Geometry: final body of the model. Coordinates: model frame, mm. A direction names the side the tool comes from. Give positions to 0.01 mm unless a question says otherwise; leave off trailing zeros. Order: outer loops, then holes, each group sorted by start corner. A loop starts at its lowest first (then second) coordinate and runs counter-clockwise, first axis right, second up. Notation, with made-up numbers: (39.25, 39.25) - (94.25, 39.25) arc R32 cw to (94.25, 68.25) - close; hole circle Ø5 at (13, 77.25). An arc over 180 degrees is marked (long way). Use one line per item in the form item = value.
Autodesk Inventor part; units mm, degrees
ref_plane "Work Plane1" through (19.939, 0, 0) normal (1, 0, 0) x (0, 0, -1)
ref_plane "fan interface" through (0, 0, 5.3975) normal (0, 0, 1) x (1, 0, 0)
ref_plane "YZ Plane" through (0, 0, 0) normal (1, 0, 0) x (0, 1, 0)
sketch "Sketch1" plane through (0, 0, 0) normal (0, 0, 1) x (1, 0, 0)
  line L0 (0, 0) -> (39.878, 0)
  line L1 (39.878, 0) -> (39.878, 39.878)
  line L2 (39.878, 39.878) -> (0, 39.878)
  line L3 (0, 39.878) -> (0, 0)
  dimension "d0" = 39.878
  dimension "d1" = 39.878
extrude "Extrusion1" add sketch "Sketch1" along normal blind 19.812
ref_plane "Work Plane1" through (19.939, 0, 0) normal (1, 0, 0) x (0, 0, -1)
sketch "Sketch2" plane through (19.939, 0, 0) normal (1, 0, 0) x (0, 0, -1)
  line L0 (-19.812, 39.878) -> (-19.812, 0)
  line L1 (0, 0) -> (0, 39.878)
  line L2 (-19.812, 19.939) -> (0, 19.939)
  line L3 (-18.1102, 52.578) -> (-1.7018, 52.578)
  line L4 (-1.7018, 52.578) -> (-1.7018, 39.878)
  line L5 (-1.7018, 39.878) -> (-18.1102, 39.878)
  line L6 (-18.1102, 39.878) -> (-18.1102, 52.578)
  line L7 (-19.812, 39.878) -> (0, 39.878)
  dimension "d4" = 1.7018
  dimension "d5" = 1.7018
  dimension "d6" = 12.7
revolve "Revolution1" cut sketch "Sketch2" angle 360 about axis through (19.939, 19.939, 19.812) along (0, 0, -1) contours L6 L3 L4 L5
fillet "Fillet1" radius 3.175 7 edges at (39.878, 39.878, 18.9611) (39.878, 39.878, 0.8509) (0, 39.878, 18.9611) (0, 39.878, 0.8509) (0, 0, 0.8509) (39.878, 0, 0.8509) (39.878, 0, 18.9611)
sketch "Sketch3" plane through (0, 0, 19.812) normal (0, 0, 1) x (1, 0, 0)
  arc A0 (39.878, 36.703) -> (36.703, 39.878) centre (36.703, 36.703) ccw
  circle A1 centre (36.703, 36.703) radius 2.286
  dimension "d9" = 4.572
extrude "Extrusion2" cut sketch "Sketch3" against normal through all
sketch "Sketch4" plane through (19.939, 39.878, 1.7018) normal (0, 0, 1) x (1, 0, 0)
  circle A0 centre (16.764, -3.175) radius 2.286
  arc A1 (19.939, -3.175) -> (16.764, 0) centre (16.764, -3.175) ccw
  arc A2 (19.939, -19.939) -> (0, 0) centre (0, -19.939) ccw
  line L0 (16.764, -3.175) -> (0, -19.939)
  circle A3 centre (16.764, -3.175) radius 2.7094
  line L1 (18.6798, -5.0908) -> (15.8841, -7.8866)
  line L2 (14.8482, -1.2592) -> (12.0524, -4.0549)
extrude "Extrusion3" add sketch "Sketch4" along normal up to next
pattern_circular "Circular Pattern1" count 4 over 360 about axis through (19.939, 19.939, 9.906) along (0, 0, 1) of "Extrusion2", "Extrusion3"
sketch "Sketch5" plane through (0, 0, 19.812) normal (0, 0, 1) x (1, 0, 0)
  arc A0 (19.939, 39.878) -> (7.8866, 35.8231) centre (19.939, 19.939) ccw
  arc A1 (31.9914, 35.8231) -> (19.939, 39.878) centre (19.939, 19.939) ccw
  arc A2 (31.9914, 35.8231) -> (19.939, 39.878) centre (19.939, 19.939) ccw
  arc A3 (19.939, 39.878) -> (7.8866, 35.8231) centre (19.939, 19.939) ccw
  circle A4 centre (19.939, 19.939) radius 19.2405
  dimension "d19" = 38.481
extrude "Extrusion4" cut sketch "Sketch5" against normal through all
sketch "Sketch6" plane through (0, 0, 0) normal (0, 0, -1) x (-1, 0, 0)
  circle A0 centre (-19.939, 19.939) radius 19.2405
  circle A1 centre (-36.703, 3.175) radius 2.286
  line L0 (-15.6996, 8.562) -> (-35.9048, 1.0329)
  line L1 (-19.5524, 7.804) -> (-34.6449, 2.18)
  line L2 (-12.546, 29.5698) -> (-0.7061, 20.4811)
  line L3 (-9.8588, 26.7065) -> (-0.7003, 19.6761)
  arc A2 (-12.546, 29.5698) -> (-19.5524, 7.804) centre (-19.939, 19.939) ccw
  arc A3 (-15.6996, 8.562) -> (-9.8588, 26.7065) centre (-19.939, 19.939) ccw
  dimension "d21" = 0.635
  dimension "d23" = 0.635
extrude "fan support1" add sketch "Sketch6" against normal blind 3.81 contours A0 L3 A3 L0 L1 A2 L2 | A0 L0 A1 L1
sketch "Sketch7" plane through (0, 0, 0) normal (0, 0, -1) x (-1, 0, 0)
  arc A0 (-12.546, 29.5698) -> (-19.5524, 7.804) centre (-19.939, 19.939) ccw
  arc A1 (-0.7061, 20.4811) -> (-30.3715, 3.7724) centre (-19.939, 19.939) ccw
  line L0 (-36.703, 39.878) -> (-3.175, 39.878)
  line L1 (-39.878, 3.175) -> (-39.878, 36.703)
  line L2 (-33.4114, 39.878) -> (-33.4114, 23.4993)
  line L3 (-28.3314, 39.878) -> (-28.3314, 29.7703)
  line L4 (-19.939, 19.939) -> (-32.8458, 27.844)
  line L5 (-33.4114, 23.4993) -> (-31.8038, 22.5147)
  line L6 (-28.3314, 29.7703) -> (-27.625, 29.3377)
  dimension "d26" = 5.08
  dimension "d27" = 8.001
  dimension "d28" = 4.0005
extrude "fan support2" add sketch "Sketch7" against normal blind 1.5875
sketch "Sketch8" plane through (0, 0, 0) normal (0, 0, -1) x (-1, 0, 0)
  line L0 (-33.4114, 33.6755) -> (-33.4114, 23.4993)
  line L1 (-33.4114, 23.4993) -> (-31.8038, 22.5147)
  line L2 (-28.3314, 29.7703) -> (-28.3314, 37.2527)
  line L3 (-36.703, 39.878) -> (-3.175, 39.878)
  line L4 (0, 36.703) -> (0, 3.175)
  arc A0 (-15.6996, 8.562) -> (-9.8588, 26.7065) centre (-19.939, 19.939) ccw
  line L5 (-31.0281, 22.7842) -> (-32.7764, 23.855)
  line L6 (-32.7764, 23.855) -> (-32.7764, 39.243)
  line L7 (-32.7764, 39.243) -> (-28.9664, 39.243)
  circle A1 centre (-19.939, 19.939) radius 11.4483
  line L8 (-28.9664, 39.243) -> (-28.9664, 26.9796)
  dimension "d31" = 22.8966
  dimension "d32" = 0.635
  dimension "d33" = 0.635
  dimension "d34" = 0.635
  dimension "d35" = 0.635
extrude "fan support3" cut sketch "Sketch8" against normal blind 1.27 contours L5 L6 L7 L8 A1
sketch "Sketch9" plane through (0, 0, 1.27) normal (0, 0, -1) x (-1, 0, 0)
  line L0 (-32.7764, 39.243) -> (-32.7764, 23.855)
  line L1 (-32.7764, 37.9276) -> (-28.9664, 37.9276)
  line L2 (-28.9664, 37.9276) -> (-28.9664, 40.5886)
  line L3 (-28.9664, 40.5886) -> (-32.7764, 40.5886)
  line L4 (-32.7764, 40.5886) -> (-32.7764, 37.9276)
extrude "fan support4" cut sketch "Sketch9" against normal blind 1.5557
sketch "Sketch10" plane through (0, 0, 0) normal (0, 0, -1) x (-1, 0, 0)
  line L0 (-32.7764, 39.243) -> (-28.9664, 39.243)
  line L1 (-36.703, 39.878) -> (-3.175, 39.878)
  line L2 (-31.1757, 39.878) -> (-29.8511, 39.878)
  line L3 (-29.8511, 39.878) -> (-29.8511, 39.243)
  line L4 (-29.8511, 39.243) -> (-31.1757, 39.243)
  line L5 (-31.1757, 39.243) -> (-31.1757, 39.878)
extrude "fan support5" cut sketch "Sketch10" against normal blind 1.5557
ref_plane "fan interface" through (0, 0, 5.3975) normal (0, 0, 1) x (1, 0, 0)
equation "\"d5\" = d4"
equation "\"d28\" = 0.5 * d27"
equation "\"d33\" = d32"
equation "\"d34\" = d33"
equation "\"d35\" = d34"
properties part number "fan body"
(1) Pull-direction query (X, two-part tool) for faces 5 (the face through (39.878, 20, 19)), 6 (the face through (6.47, 2.64, 9.79)), 7 (the face through (37.3, 32.8, 18.11)), 8 (the face through (20, 20, 0)); classes: released by +X, released by -X, zero draft, split by the parting line, or undercut.
Computed values:
face_5 = released by +X
face_6 = undercut
face_7 = undercut
face_8 = zero draft
(2) Cut plane C-C on y = 30.5. Output: boundary loops of the cut face in (x, z), plus the area to 3 significant figures.
Computed values:
outline = (0, 0) - (3.86, 0) - (3.86, 19.81) - (0, 19.81) - (0, 18.11) - (3.03, 18.11) - (3.03, 1.7) - (0, 1.7) - close; (13.95, 0) - (25.93, 0) - (25.93, 3.81) - (13.95, 3.81) - close; (28.33, 0) - (28.97, 0) - (28.97, 1.27) - (32.78, 1.27) - (32.78, 0) - (33.41, 0) - (33.41, 1.59) - (28.33, 1.59) - close; (36.02, 0) - (39.88, 0) - (39.88, 1.7) - (36.85, 1.7) - (36.85, 18.11) - (39.88, 18.11) - (39.88, 19.81) - (36.02, 19.81) - close
area = 102 mm²
(3) Ray query, line 1 along X through (y, z) = (5, 18); line 2 along X through (y, z) = (3.5, 6.5); line 3 along Z through (x, y) = (28, 18.5). Return the intervals inside material, ascending.
Computed values:
line_1 = 1.17 to 1.8, 4.55 to 7.81, 32.06 to 35.33, 38.08 to 38.71
line_2 = 0.49 to 0.91, 5.44 to 7.33, 8.66 to 9.94, 29.94 to 31.22, 32.55 to 34.44, 38.97 to 39.39
line_3 = 0 to 3.81
(4) Reachability of faces 1 (the face through (2.6, 32.8, 18.11)), 2 (the face through (0.91, 0.95, 0.86)), 3 (the face through (2.637, 33.409, 9.791)), 4 (the face through (33.41, 37.24, 9.79)) from +Z, -Z, +X, -X, +Y, -Y: full face, straight path, thin tool, end or side. Return the list, or none.
Computed values:
face_1 = none
face_2 = -Z, -X, -Y
face_3 = -X
face_4 = +Y
(5) Cut plane A-A on y = 6. Output: boundary loops of the cut face in (x, z).
Computed values:
outline = (0, 0) - (6.68, 0) - (6.68, 19.81) - (0, 19.81) - (0, 18.11) - (2.17, 18.11) - (2.17, 1.7) - (0, 1.7) - close; (22.58, 0) - (24.39, 0) - (24.39, 3.81) - (22.58, 3.81) - close; (33.2, 0) - (39.88, 0) - (39.88, 1.7) - (37.71, 1.7) - (37.71, 18.11) - (39.88, 18.11) - (39.88, 19.81) - (33.2, 19.81) - close
(6) Cut plane D-D on z = 17.25. Output: boundary loops of the cut face in (x, y) (1 decimal), plus the area to 3 significant figures.
Computed values:
outline = (1.3, 5.1) arc R2.7 ccw to (5.1, 1.3) - (7.9, 4.1) arc R19.9 ccw to (32, 4.1) - (34.8, 1.3) arc R2.7 ccw to (38.6, 5.1) - (35.8, 7.9) arc R19.9 ccw to (35.8, 32) - (38.6, 34.8) arc R2.7 ccw to (34.8, 38.6) - (32, 35.8) arc R19.9 ccw to (7.9, 35.8) - (5.1, 38.6) arc R2.7 ccw to (1.3, 34.8) - (4.1, 32) arc R19.9 ccw to (4.1, 7.9) - close; hole circle Ø38.5 at (19.9, 19.9); hole circle Ø4.6 at (3.2, 3.2); hole circle Ø4.6 at (3.2, 36.7); hole circle Ø4.6 at (36.7, 3.2); hole circle Ø4.6 at (36.7, 36.7)
area = 149 mm²
(7) Cut plane B-B on x = 17. Output: boundary loops of the cut face in (y, z), plus the area to 3 significant figures.
Computed values:
outline = (0, 0) - (0.92, 0) - (0.92, 19.81) - (0, 19.81) - (0, 18.11) - (0.22, 18.11) - (0.22, 1.7) - (0, 1.7) - close; (8.08, 0) - (31.72, 0) - (31.72, 3.81) - (8.08, 3.81) - close; (38.95, 0) - (39.88, 0) - (39.88, 1.7) - (39.66, 1.7) - (39.66, 18.11) - (39.88, 18.11) - (39.88, 19.81) - (38.95, 19.81) - close
area = 120 mm²
(8) Contact query for flat-ended pins moving along their axis: pin 1 Ø2 at (x, z) = (7.5, 8.5) entering from +Y; pin 2 Ø3 at (x, y) = (13, 20) entering from +Z; pin 3 Ø2 at (y, z) = (16.5, 5.5) entering from -X. Output: stop coordinate, or through.
Computed values:
pin_1 = 37.21
pin_2 = 3.81
pin_3 = 0.15
